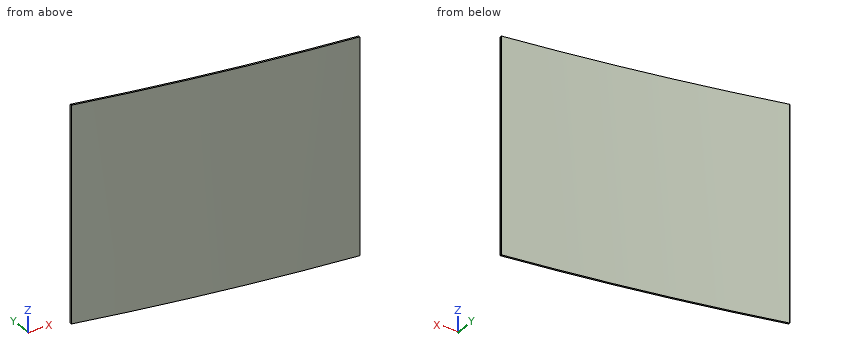
from build123d import *

# Parameters (mm, degrees)
BOSS_EXTRUDE1_DEPTH = 600


with BuildPart() as part:
    # Sketch2 → Boss-Extrude1 (new body)
    with BuildSketch(Plane.XY):
        with BuildLine():
            Line((8671.180248107, -15050.67644099), (8671.180248107, -15047.570291511))
            ThreePointArc((8671.180248107, -15047.570291511), (8296.961694468, -15002.727582577), (7925.803525446, -14937.214164091))
            Line((7925.803525446, -14937.214164091), (7924.798244697, -14937.007753794))
            Line((7924.798244697, -14937.007753794), (7924.798244697, -14942.112062683))
            ThreePointArc((7924.798244697, -14942.112062683), (8296.455606532, -15007.707153296), (8671.178621007, -15052.591147568))
            Line((8671.178621007, -15052.591147568), (8671.180248107, -15050.67644099))
        make_face()
    extrude(amount=BOSS_EXTRUDE1_DEPTH)


solid = part.part
Work out the finished part from the listing and answer in its coordinate system (mm). Round coordinates to 2 decimals unless told otherwise and drop trailing zeros. Write each loop counter-clockwise with the first axis right and the second up, starting at its lowest first coordinate (ties: lowest second). Pieces come first, ordered by that corner, then holes. Notation, with made-up numbers: (-38.5, -2) - (18.5, -2) arc R23 ccw to (18.5, 35) - close; hole circle Ø7 at (-35, 86.25). An arc over 180 degrees is marked (long way). Answer in a Markdown table with one row per item. Add a question column.
1. A cutting plane is placed at C-C, the plane x = 8512. Determine the outline of the cut face in (y, z), and give its area (3 significant figures).
2. Given pin 1 (3 mm diameter, centred on x = 8009, z = 221, fed in from -Y); pin 2 (10 mm diameter, centred on x = 8120, y = -14965.5, fed in from -Z), each flat-ended and moving along its own axis, determine where each tip first touches the part or whether it passes through.
3. Find the intervals of material crossed by line 1 along Y through (x, z) = (8596.5, 321); line 2 along Y through (x, z) = (8637.5, 245.5), in increasing order. Write a range as from..to.
4. A cutting plane is placed at A-A, the plane z = 442. Determine the outline of the cut face in (x, y).
Worked out:
| question | item | result |
|---|---|---|
| 1 | outline | (-15036.1, 0) - (-15031.07, 0) - (-15031.07, 600) - (-15036.1, 600) - close |
| 1 | area | 3,020 mm^2 |
| 2 | pin 1 | y = -14959.13 |
| 2 | pin 2 | through |
| 3 | line 1 | -15045.33..-15040.3 |
| 3 | line 2 | -15049.42..-15044.39 |
| 4 | outline | (7924.8, -14942.11) arc R6802.96 ccw to (8671.18, -15052.59) - (8671.18, -15050.68) - (8671.18, -15047.57) arc R6797.96 cw to (7925.8, -14937.21) - (7924.8, -14937.01) - close |
